Verification items for the finished model (mm, model axes). Face numbers are marked on the shaded views. Give positions to 0.01 mm unless a question says otherwise; leave off trailing zeros. Write each loop counter-clockwise with the first axis right and the second up, starting at its lowest first coordinate (ties: lowest second). Pieces come first, ordered by that corner, then holes. Notation, with made-up numbers: (-39, -31.75) -> (-2, -31.75) arc R22 cw to (-2, -16.75) -> close; hole circle Ø4 at (48, 81.25). An arc over 180 degrees is marked (long way). Answer as CSV lines item,"result".
```python
from build123d import *

# Parameters (mm, degrees)
SKIZZE1_W                                 = 184
SKIZZE1_H                                 = 180
EXTRUSION1_DEPTH                          = 200
SKIZZE2_R                                 = 75
EXTRUSION2_DEPTH                          = 18.5
SKIZZE3_R                                 = 75
EXTRUSION3_DEPTH                          = 16.5
M6_GEWINDEBOHRUNG1_AT_2_COUNT             = 2
M6_GEWINDEBOHRUNG1_AT_2_PITCH             = 29.520190203
SKIZZE6_R                                 = 71
EXTRUSION4_DEPTH                          = 180
FASE1_SIZE                                = 2
LINEARES_MUSTER111_COUNT                  = 3
LINEARES_MUSTER111_PITCH                  = 80
LINEARES_MUSTER111_COUNT_DIR2             = 2
LINEARES_MUSTER111_PITCH_DIR2             = 130
KREISMUSTER1_COUNT                        = 4
M6_GEWINDEBOHRUNG2_AT_2_COUNT             = 2
M6_GEWINDEBOHRUNG2_AT_2_PITCH             = 31.25667198
KREISMUSTER2_COUNT                        = 4
F_16_0_16_DURCHMESSER_BOHRUNG1_AT_2_COUNT = 2
F_16_0_16_DURCHMESSER_BOHRUNG1_AT_2_PITCH = 170.293863659
M5_GEWINDEBOHRUNG1_D                      = 4.2
M5_GEWINDEBOHRUNG1_DEPTH                  = 10
M5_GEWINDEBOHRUNG1_TIP                    = 1.2618073


with BuildPart() as part:
    # Skizze1 → Extrusion1 (new body)
    with BuildSketch(Plane.XY):
        Rectangle(SKIZZE1_W, SKIZZE1_H)
    extrude(amount=EXTRUSION1_DEPTH)

    # Skizze2 → Extrusion2 (cut)
    with BuildSketch(Plane.XY.offset(200)):
        Circle(SKIZZE2_R)
    extrude(amount=-EXTRUSION2_DEPTH, mode=Mode.SUBTRACT)

    # Skizze3 → Extrusion3 (cut)
    with BuildSketch(Plane(origin=(0, 0, 0), x_dir=(-1, 0, 0), z_dir=(0, 0, -1))):
        with Locations(Location((0, 0, 0), (0, 0, 180))):  # turned: the seam where the file's is
            Circle(SKIZZE3_R)
    extrude(amount=-EXTRUSION3_DEPTH, mode=Mode.SUBTRACT)

    # Skizze10 → M6 Gewindebohrung1 (revolve, cut)
    with BuildSketch(Plane(origin=(69.627923765, 48.75399709, 0), x_dir=(0, 1, 0), z_dir=(1, 0, 0))):
        Polygon((0, 0), (0, 18.502151548), (2.5, 17), (2.5, 0), align=None)
    m6_gewindebohrung1 = revolve(axis=Axis((69.627923765, 48.75399709, -6.35), (0, 0, 1)), mode=Mode.SUBTRACT)

    # M6 Gewindebohrung1 at 2: M6 Gewindebohrung1 ×2
    with Locations(*[Vector(-0.707106781, 0.707106781, 0) * (i * M6_GEWINDEBOHRUNG1_AT_2_PITCH) for i in range(1, M6_GEWINDEBOHRUNG1_AT_2_COUNT)]):
        add(m6_gewindebohrung1, mode=Mode.SUBTRACT)

    # Skizze6 → Extrusion4 (cut)
    with BuildSketch(Plane(origin=(0, 0, 16.5), x_dir=(-1, 0, 0), z_dir=(0, 0, -1))):
        Circle(SKIZZE6_R)
    extrude(amount=-EXTRUSION4_DEPTH, mode=Mode.SUBTRACT)

    # Fase1
    fase1_edges = [part.edges().sort_by_distance(p)[0] for p in [
        (92, 0, 200),
        (0, 90, 200),
        (-92, 0, 200),
        (0, 90, 0),
        (92, 0, 0),
        (0, -90, 0),
        (-92, 0, 0),
        (0, -90, 200),
        (-92, 90, 100),
        (92, 90, 100),
        (92, -90, 100),
        (-92, -90, 100),
    ]]
    chamfer(fase1_edges, length=FASE1_SIZE)

    # Skizze14 → M16 Gewindebohrung3 (revolve, cut)
    with BuildSketch(Plane(origin=(-92, 65, 180), x_dir=(0, 0, 1), z_dir=(0, 1, 0))):
        Polygon((0, 0), (0, 42.206024333), (7, 38), (7, 0), align=None)
    m16_gewindebohrung3 = revolve(axis=Axis((-98.35, 65, 180), (1, 0, 0)), mode=Mode.SUBTRACT)

    # Lineares Muster111: M16 Gewindebohrung3 3 × 2
    with Locations(*[(0, -j * LINEARES_MUSTER111_PITCH_DIR2, -i * LINEARES_MUSTER111_PITCH) for i in range(LINEARES_MUSTER111_COUNT) for j in range(LINEARES_MUSTER111_COUNT_DIR2) if (i, j) != (0, 0)]):
        add(m16_gewindebohrung3, mode=Mode.SUBTRACT)

    # Spiegeln3: M16 Gewindebohrung3 across plane
    add(m16_gewindebohrung3.mirror(Plane(origin=(0, 0, 0), x_dir=(0, 0, 1), z_dir=(1, 0, 0))), mode=Mode.SUBTRACT)

    # Spiegeln3 copy 1 sketch → Spiegeln3 copy 1 (revolve, cut)
    with BuildSketch(Plane(origin=(92, -65, 180), x_dir=(0, 0, 1), z_dir=(0, 1, 0))):
        Polygon((0, 0), (0, -42.206024333), (7, -38), (7, 0), align=None)
    revolve(axis=Axis((98.35, -65, 180), (1, 0, 0)), mode=Mode.SUBTRACT)

    # Spiegeln3 copy 2 sketch → Spiegeln3 copy 2 (revolve, cut)
    with BuildSketch(Plane(origin=(92, 65, 100), x_dir=(0, 0, 1), z_dir=(0, 1, 0))):
        Polygon((0, 0), (0, -42.206024333), (7, -38), (7, 0), align=None)
    revolve(axis=Axis((98.35, 65, 100), (1, 0, 0)), mode=Mode.SUBTRACT)

    # Spiegeln3 copy 3 sketch → Spiegeln3 copy 3 (revolve, cut)
    with BuildSketch(Plane(origin=(92, -65, 100), x_dir=(0, 0, 1), z_dir=(0, 1, 0))):
        Polygon((0, 0), (0, -42.206024333), (7, -38), (7, 0), align=None)
    revolve(axis=Axis((98.35, -65, 100), (1, 0, 0)), mode=Mode.SUBTRACT)

    # Spiegeln3 copy 4 sketch → Spiegeln3 copy 4 (revolve, cut)
    with BuildSketch(Plane(origin=(92, 65, 20), x_dir=(0, 0, 1), z_dir=(0, 1, 0))):
        Polygon((0, 0), (0, -42.206024333), (7, -38), (7, 0), align=None)
    revolve(axis=Axis((98.35, 65, 20), (1, 0, 0)), mode=Mode.SUBTRACT)

    # Spiegeln3 copy 5 sketch → Spiegeln3 copy 5 (revolve, cut)
    with BuildSketch(Plane(origin=(92, -65, 20), x_dir=(0, 0, 1), z_dir=(0, 1, 0))):
        Polygon((0, 0), (0, -42.206024333), (7, -38), (7, 0), align=None)
    revolve(axis=Axis((98.35, -65, 20), (1, 0, 0)), mode=Mode.SUBTRACT)

    # Kreismuster1: M6 Gewindebohrung1 ×4 about axis
    kreismuster1_axis = Axis((0, 0, 0), (0, 0, 1))
    for i in range(1, KREISMUSTER1_COUNT):
        add(m6_gewindebohrung1.rotate(kreismuster1_axis, i * 360 / KREISMUSTER1_COUNT), mode=Mode.SUBTRACT)

    # Kreismuster1 copy 1 sketch → Kreismuster1 copy 1 (revolve, cut)
    with BuildSketch(Plane(origin=(-69.627923765, 48.75399709, 0), x_dir=(-1, 0, 0), z_dir=(0, 1, 0))):
        Polygon((0, 0), (0, 18.502151548), (2.5, 17), (2.5, 0), align=None)
    revolve(axis=Axis((-69.627923765, 48.75399709, -6.35), (0, 0, 1)), mode=Mode.SUBTRACT)

    # Kreismuster1 copy 2 sketch → Kreismuster1 copy 2 (revolve, cut)
    with BuildSketch(Plane(origin=(-48.75399709, -69.627923765, 0), x_dir=(0, -1, 0), z_dir=(-1, 0, 0))):
        Polygon((0, 0), (0, 18.502151548), (2.5, 17), (2.5, 0), align=None)
    revolve(axis=Axis((-48.75399709, -69.627923765, -6.35), (0, 0, 1)), mode=Mode.SUBTRACT)

    # Kreismuster1 copy 3 sketch → Kreismuster1 copy 3 (revolve, cut)
    with BuildSketch(Plane(origin=(69.627923765, -48.75399709, 0), x_dir=(1, 0, 0), z_dir=(0, -1, 0))):
        Polygon((0, 0), (0, 18.502151548), (2.5, 17), (2.5, 0), align=None)
    revolve(axis=Axis((69.627923765, -48.75399709, -6.35), (0, 0, 1)), mode=Mode.SUBTRACT)

    # Skizze16 → M6 Gewindebohrung2 (revolve, cut)
    with BuildSketch(Plane(origin=(-73.723683986, 51.621879272, 200), x_dir=(0, -1, 0), z_dir=(1, 0, 0))):
        Polygon((0, 0), (0, 18.502151548), (2.5, 17), (2.5, 0), align=None)
    m6_gewindebohrung2 = revolve(axis=Axis((-73.723683986, 51.621879272, 206.35), (0, 0, -1)), mode=Mode.SUBTRACT)

    # M6 Gewindebohrung2 at 2: M6 Gewindebohrung2 ×2
    with Locations(*[Vector(0.707106781, 0.707106781, 0) * (i * M6_GEWINDEBOHRUNG2_AT_2_PITCH) for i in range(1, M6_GEWINDEBOHRUNG2_AT_2_COUNT)]):
        add(m6_gewindebohrung2, mode=Mode.SUBTRACT)

    # Kreismuster2: M6 Gewindebohrung2 ×4 about axis
    kreismuster2_axis = Axis((0, 0, 0), (0, 0, 1))
    for i in range(1, KREISMUSTER2_COUNT):
        add(m6_gewindebohrung2.rotate(kreismuster2_axis, i * 360 / KREISMUSTER2_COUNT), mode=Mode.SUBTRACT)

    # Kreismuster2 copy 1 sketch → Kreismuster2 copy 1 (revolve, cut)
    with BuildSketch(Plane(origin=(-73.723683986, -51.621879272, 200), x_dir=(1, 0, 0), z_dir=(0, 1, 0))):
        Polygon((0, 0), (0, 18.502151548), (2.5, 17), (2.5, 0), align=None)
    revolve(axis=Axis((-73.723683986, -51.621879272, 206.35), (0, 0, -1)), mode=Mode.SUBTRACT)

    # Kreismuster2 copy 2 sketch → Kreismuster2 copy 2 (revolve, cut)
    with BuildSketch(Plane(origin=(51.621879272, -73.723683986, 200), x_dir=(0, 1, 0), z_dir=(-1, 0, 0))):
        Polygon((0, 0), (0, 18.502151548), (2.5, 17), (2.5, 0), align=None)
    revolve(axis=Axis((51.621879272, -73.723683986, 206.35), (0, 0, -1)), mode=Mode.SUBTRACT)

    # Kreismuster2 copy 3 sketch → Kreismuster2 copy 3 (revolve, cut)
    with BuildSketch(Plane(origin=(73.723683986, 51.621879272, 200), x_dir=(-1, 0, 0), z_dir=(0, -1, 0))):
        Polygon((0, 0), (0, 18.502151548), (2.5, 17), (2.5, 0), align=None)
    revolve(axis=Axis((73.723683986, 51.621879272, 206.35), (0, 0, -1)), mode=Mode.SUBTRACT)

    # Skizze18 → Ø16.0 (16) Durchmesser Bohrung1 (revolve, cut)
    with BuildSketch(Plane(origin=(92, 65, 155), x_dir=(0, 0, -1), z_dir=(0, 1, 0))):
        Polygon((0, 0), (0, 27.056884952), (8, 22.25), (8, 0), align=None)
    f_16_0_16_durchmesser_bohrung1 = revolve(axis=Axis((98.35, 65, 155), (-1, 0, 0)), mode=Mode.SUBTRACT)

    # Ø16.0 (16) Durchmesser Bohrung1 at 2: Ø16.0 (16) Durchmesser Bohrung1 ×2
    with Locations(*[Vector(0, -0.763386285, -0.645942241) * (i * F_16_0_16_DURCHMESSER_BOHRUNG1_AT_2_PITCH) for i in range(1, F_16_0_16_DURCHMESSER_BOHRUNG1_AT_2_COUNT)]):
        add(f_16_0_16_durchmesser_bohrung1, mode=Mode.SUBTRACT)

    # Spiegeln4: Ø16.0 (16) Durchmesser Bohrung1 across plane
    add(f_16_0_16_durchmesser_bohrung1.mirror(Plane(origin=(0, 0, 0), x_dir=(0, 0, 1), z_dir=(1, 0, 0))), mode=Mode.SUBTRACT)

    # Spiegeln4 copy 1 sketch → Spiegeln4 copy 1 (revolve, cut)
    with BuildSketch(Plane(origin=(-92, -65, 45), x_dir=(0, 0, -1), z_dir=(0, 1, 0))):
        Polygon((0, 0), (0, -27.056884952), (8, -22.25), (8, 0), align=None)
    revolve(axis=Axis((-98.35, -65, 45), (-1, 0, 0)), mode=Mode.SUBTRACT)

    # M5 Gewindebohrung1
    with Locations(Plane(origin=(0, -90, 0), x_dir=(-1, 0, 0), z_dir=(0, -1, 0))):
        with Locations((-40, -180), (-18, -180)):
            Hole(M5_GEWINDEBOHRUNG1_D / 2, depth=M5_GEWINDEBOHRUNG1_DEPTH)
            with Locations((0, 0, -(M5_GEWINDEBOHRUNG1_DEPTH + M5_GEWINDEBOHRUNG1_TIP / 2))):  # 118° drill point
                Cone(0, M5_GEWINDEBOHRUNG1_D / 2, M5_GEWINDEBOHRUNG1_TIP, mode=Mode.SUBTRACT)


solid = part.part
```
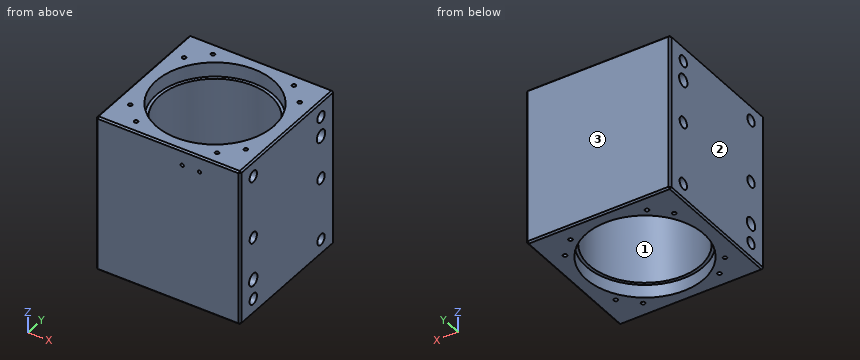
1) Scan lines: line 1 along Z through (x, y) = (-82.25, 65); line 2 along Y through (x, z) = (82, 20); line 3 along Z through (x, y) = (69, 65). Record each from-to range of solid material in increasing order.
Reported:
line 1,"0 to 13, 27 to 93, 107 to 147, 163 to 173, 187 to 200"
line 2,"-90 to -72, -58 to 58, 72 to 90"
line 3,"0 to 13, 27 to 93, 107 to 148.25, 161.75 to 173, 187 to 200"
2) Section check B-B (x = 0). Record the boundary of the cut face in (y, z).
Reported:
outline,"(-90, 2) -> (-88, 0) -> (-75, 0) -> (-75, 16.5) -> (-71, 16.5) -> (-71, 181.5) -> (-75, 181.5) -> (-75, 200) -> (-88, 200) -> (-90, 198) -> close; (71, 16.5) -> (75, 16.5) -> (75, 0) -> (88, 0) -> (90, 2) -> (90, 198) -> (88, 200) -> (75, 200) -> (75, 181.5) -> (71, 181.5) -> close"
3) Section check A-A (z = 141.5). Record the boundary of the cut face in (x, y).
Reported:
outline,"(-92, -88) -> (-90, -90) -> (90, -90) -> (92, -88) -> (92, 88) -> (90, 90) -> (-90, 90) -> (-92, 88) -> close; hole circle Ø142 at (0, 0)"
4) Depth check by flat-ended pin: pin 1 (22.5 mm diameter, centred on y = 65, z = 180, fed in from -X); pin 2 (6 mm diameter, centred on x = -67.5, y = 4, fed in from -Z); pin 3 (11 mm diameter, centred on y = 65, z = 100, fed in from -X); pin 4 (8.5 mm diameter, centred on y = -65, z = 100, fed in from -X). Enter the tip coordinate at first touch or a pass-through.
Reported:
pin 1,"x = -92"
pin 2,"through"
pin 3,"x = -53.1"
pin 4,"x = -52.35"
5) Draft check along Y on the marked faces 1, 2 and 3. Enter one of: +Y half, -Y half, draft (parallel to the pull), parting line (faces both ways), or undercut.
Reported:
face 1,"undercut"
face 2,"draft"
face 3,"+Y half"
6) Section check C-C (x = -22). Record the boundary of the cut face in (y, z), and give its area (3 significant figures).
Reported:
outline,"(-90, 2) -> (-88, 0) -> (-71.7, 0) -> (-71.7, 16.5) -> (-67.51, 16.5) -> (-67.51, 181.5) -> (-71.7, 181.5) -> (-71.7, 200) -> (-88, 200) -> (-90, 198) -> close; (67.51, 16.5) -> (71.7, 16.5) -> (71.7, 0) -> (88, 0) -> (90, 2) -> (90, 198) -> (88, 200) -> (71.7, 200) -> (71.7, 181.5) -> (67.51, 181.5) -> close"
area,"8,700 mm²"
